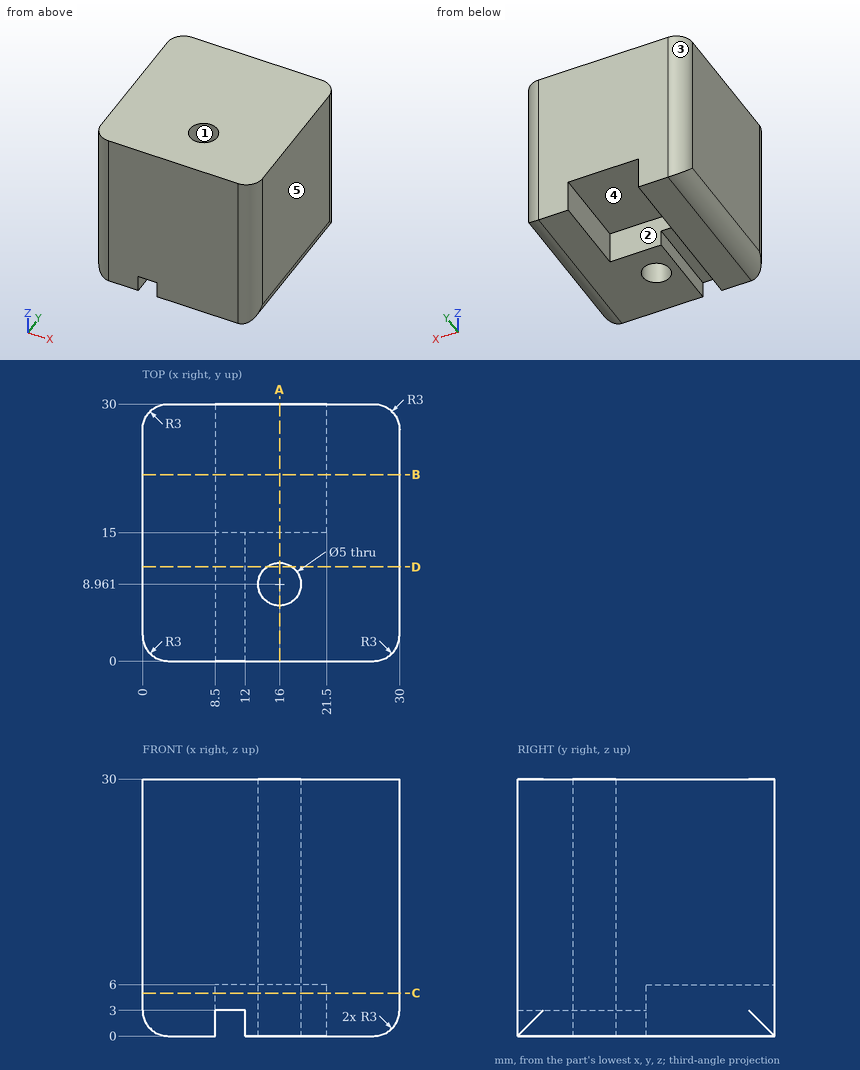
Drawing for the job (mm, zero at the part's lowest x, y, z). A direction names the side the tool comes from. Coordinates: 2 decimals unless noted, no trailing zeros. Order: outer loops, then holes, each group sorted by start corner. A loop starts at its lowest first (then second) coordinate and runs counter-clockwise, first axis right, second up.
Item 1: Pin check, flat tips, straight feed: pin 1 Ø5 at (x, z) = (17.5, 2.5) entering from +Y; pin 2 Ø0.9 at (y, z) = (4.5, 1.5) entering from -X. Stop position of each tip, or through.
Check sheet entries:
pin 1: stops at y = 15
pin 2: stops at x = 0.19
Item 2: Band-saw the part on C-C on z = 5. List the corners of the cut face in (x, y).
Check sheet entries:
outline: (0, 3) arc R3 ccw to (3, 0) - (27, 0) arc R3 ccw to (30, 3) - (30, 27) arc R3 ccw to (27, 30) - (21.5, 30) - (21.5, 15) - (8.5, 15) - (8.5, 30) - (3, 30) arc R3 ccw to (0, 27) - close; hole circle Ø5 at (16, 8.96)
Item 3: Band-saw the part on B-B on y = 21.75. List the corners of the cut face in (x, z), plus the area to 3 significant figures.
Check sheet entries:
outline: (0, 3) arc R3 ccw to (3, 0) - (8.5, 0) - (8.5, 6) - (21.5, 6) - (21.5, 0) - (27, 0) arc R3 ccw to (30, 3) - (30, 30) - (0, 30) - close
area: 818 mm2
Item 4: Band-saw the part on A-A on x = 16. List the corners of the cut face in (y, z).
Check sheet entries:
outline: (0, 0) - (6.46, 0) - (6.46, 30) - (0, 30) - close; (11.46, 0) - (15, 0) - (15, 6) - (30, 6) - (30, 30) - (11.46, 30) - close
Item 5: 3-axis set-ups, long thin cutter, end or side, ignore diameter. For the marked faces 1 and 2: which of +Z, -Z, +X, -X, +Y, -Y reach the whole face in a straight line?
Check sheet entries:
face 1: +Z, -Z
face 2: -Z, +Y
Item 6: Band-saw the part on D-D on y = 11. List the corners of the cut face in (x, z).
Check sheet entries:
outline: (0, 3) arc R3 ccw to (3, 0) - (8.5, 0) - (8.5, 3) - (12, 3) - (12, 0) - (14.55, 0) - (14.55, 30) - (0, 30) - close; (17.45, 0) - (27, 0) arc R3 ccw to (30, 3) - (30, 30) - (17.45, 30) - close
Item 7: Drill centre lines: L1, parallel to Y at x = 16, z = 9.75; L2, parallel to Y at x = 16.5, z = 23; L3, parallel to Z at x = 27.25, y = 15.75. Where is each one in solid material? Low to high.
Check sheet entries:
L1: y = 0 to 6.46, 11.46 to 30
L2: y = 0 to 6.51, 11.41 to 30
L3: z = 0.01 to 30
Item 8: Two-plate mould, pull along X, no slides. Class the marked faces 3, 4 and 5: +X half, -X half, draft (parallel to the pull), parting line (faces both ways), or undercut.
Check sheet entries:
face 3: -X half
face 4: undercut
face 5: +X half
